Input: part model. Units: mm. Frame: model coordinates. Face numbers are marked on the shaded views. A direction names the side the tool comes from. Coordinates: 2 decimals unless noted, no trailing zeros. Write each loop counter-clockwise with the first axis right and the second up, starting at its lowest first coordinate (ties: lowest second). Pieces come first, ordered by that corner, then holes. Notation, with made-up numbers: (33.25, 56.25) - (83.25, 56.25) arc R14 cw to (83.25, 63.25) - close; hole circle Ø11 at (78.5, 64.25). An arc over 180 degrees is marked (long way). Use a Markdown table: item, result. Add a question column.
Q1. Section query D-D (z = 13.5). Return the cut outline in (x, y), then the cut area to 3 significant figures.
Q2. Pin query (flat end, axial travel): P1, Ø5, axis at x = 0, z = 19.5, coming from the +Y side; P2, Ø1, axis at x = -13.5, y = 9, coming from the +Z side (3 decimals). Return the tip coordinate at first contact, or that it passes through.
Q3. Mould query, pull axis X, two halves, no side actions, for the marked faces 3, 4, 5 and 6. Classes: released by +X, released by -X, zero draft, split by the parting line, or undercut.
Q4. Section query C-C (y = 8). Return the cut outline in (x, z) (3 decimals).
Q5. Section query A-A (x = -9). Return the cut outline in (y, z) (3 decimals), then the cut area to 3 significant figures.
Q6. Set-up query: the marked faces 1 and 2. Return all of +Z, -Z, +X, -X, +Y, -Y with unobstructed straight access to the full face (end or side cutting, diameter ignored); none if empty.
Q7. Section query B-B (x = -2.5). Return the cut outline in (y, z) (3 decimals), then the cut area to 3 significant figures.
Q8. Material intervals for probe 1 along Z at (x, y) = (-0.5, 0.25) (3 decimals); probe 2 along Y at (x, z) = (-2.25, 20.75); probe 3 along X at (y, z) = (-7, 14.75), sorted ascending. Write a range as from..to.
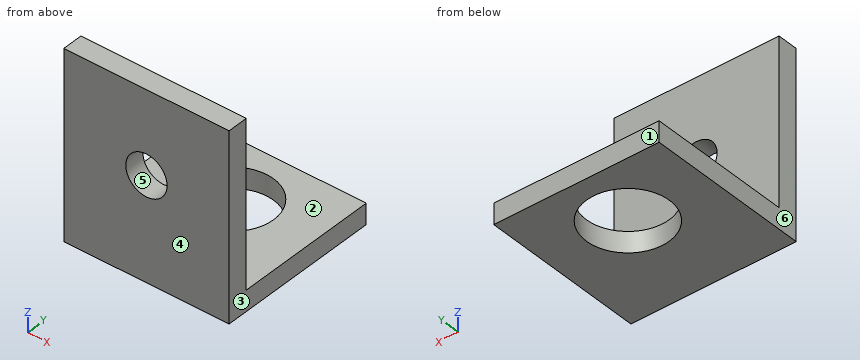
Autodesk Inventor part; units mm, degrees
ref_plane "YZ Plane" through (0, 0, 0) normal (1, 0, 0) x (0, 1, 0)
ref_plane "XZ Plane" through (0, 0, 0) normal (0, 1, 0) x (-1, 0, 0)
ref_plane "XY Plane" through (0, 0, 0) normal (0, 0, 1) x (1, 0, 0)
sketch "Sketch1" plane through (0, 0, 0) normal (0, 0, 1) x (1, 0, 0)
  line L0 (9.1118, -9.9057) -> (-16.2882, -9.9057)
  line L1 (-16.2882, -9.9057) -> (-16.2882, 15.4943)
  line L2 (-16.2882, 15.4943) -> (9.1118, 15.4943)
  line L3 (9.1118, 15.4943) -> (9.1118, -9.9057)
  circle A0 centre (-3.5882, 5.9693) radius 6.35
  point P0 (0, 0)
  dimension "d0" = 25.4
  dimension "d1" = 25.4
  dimension "d2" = 12.7
  dimension "d16" = 9.525
extrude "Extrusion1" add sketch "Sketch1" along normal blind 3.175
sketch "Sketch2" plane through (0, 0, 3.175) normal (0, 0, 1) x (1, 0, 0)
  line L0 (9.1118, 15.4943) -> (9.1118, -9.9057)
  line L1 (-16.2882, -9.9057) -> (9.1118, -9.9057)
  line L2 (9.1118, -9.9057) -> (9.1118, -6.7307)
  line L3 (9.1118, -6.7307) -> (-16.2882, -6.7307)
  line L4 (-16.2882, -6.7307) -> (-16.2882, -9.9057)
  point P0 (0, 0)
  dimension "d5" = 3.175
extrude "Extrusion2" add sketch "Sketch2" along normal blind 25.4
sketch "Sketch3" plane through (-16.2882, -6.7307, 3.175) normal (0, 1, 0) x (1, 0, 0)
  line L0 (0, -25.4) -> (25.4, -25.4)
  line L1 (25.4, 0) -> (25.4, -25.4)
  circle A0 centre (12.7, -12.7) radius 3.175
  point P0 (16.2882, 3.175)
  dimension "d9" = 6.35
  dimension "d11" = 12.7
  dimension "d13" = 12.7
extrude "Extrusion3" cut sketch "Sketch3" against normal blind 25.4
properties part number "Piston Mounting Bracket"
Values follow:
| question | item | result |
|---|---|---|
| 1 | outline | (-16.29, -9.91) - (-5.7, -9.91) - (-5.7, -6.73) - (-16.29, -6.73) - close; (-1.48, -9.91) - (9.11, -9.91) - (9.11, -6.73) - (-1.48, -6.73) - close |
| 1 | area | 67.3 mm2 |
| 2 | P1 | y = -6.73 |
| 2 | P2 | z = 3.175 |
| 3 | face 3 | released by +X |
| 3 | face 4 | zero draft |
| 3 | face 5 | undercut |
| 3 | face 6 | released by -X |
| 4 | outline | (-16.288, 0) - (-9.605, 0) - (-9.605, 3.175) - (-16.288, 3.175) - close; (2.428, 0) - (9.112, 0) - (9.112, 3.175) - (2.428, 3.175) - close |
| 5 | outline | (-9.906, 0) - (2.647, 0) - (2.647, 3.175) - (-6.731, 3.175) - (-6.731, 28.575) - (-9.906, 28.575) - close; (9.291, 0) - (15.494, 0) - (15.494, 3.175) - (9.291, 3.175) - close |
| 5 | area | 140 mm2 |
| 6 | face 1 | +Z, -Z, +X, -X, +Y |
| 6 | face 2 | +Z, +X, -X, +Y |
| 7 | outline | (-9.906, 0) - (-0.287, 0) - (-0.287, 3.175) - (-6.731, 3.175) - (-6.731, 12.892) - (-9.906, 12.892) - close; (-9.906, 18.858) - (-6.731, 18.858) - (-6.731, 28.575) - (-9.906, 28.575) - close; (12.225, 0) - (15.494, 0) - (15.494, 3.175) - (12.225, 3.175) - close |
| 7 | area | 103 mm2 |
| 8 | probe 1 | 0..3.175 |
| 8 | probe 2 | -9.91..-6.73 |
| 8 | probe 3 | -16.29..-6.56, -0.62..9.11 |
